from build123d import *

# Parameters (mm, degrees)
BOSS_EXTRUDE1_DEPTH      = 5.1
BOSS_EXTRUDE1_DEPTH_BACK = 5.1
SKETCH1_W                = 18
SKETCH1_H                = 15
SKETCH1_R                = 2.1
CUT_EXTRUDE1_DEPTH       = 4.1
CUT_EXTRUDE1_DEPTH_BACK  = 4.1
SKETCH4_W                = 6.8
SKETCH4_H                = 7.2
CUT_EXTRUDE2_DEPTH       = 7.5
SKETCH6_R                = 4.9
CUT_EXTRUDE4_DEPTH       = 4.5
SKETCH7_R                = 7.5
SKETCH7_R_2              = 3.225
BOSS_EXTRUDE2_DEPTH      = 1
SKETCH8_W                = 7.5
SKETCH8_H                = 2.6
CUT_EXTRUDE5_DEPTH       = 6.5


with BuildPart() as part:
    # Sketch1 → Boss-Extrude1 (new, two sides: drawn at the far end of the back side and taken through both)
    with BuildSketch(Plane(origin=(0, 0, 0), x_dir=(1, 0, 0), z_dir=(0, 1, 0)).offset(-BOSS_EXTRUDE1_DEPTH_BACK)):
        Rectangle(SKETCH1_W, SKETCH1_H)
        with Locations(Location((0, 0, 0), (0, 0, 270))):
            Circle(SKETCH1_R, mode=Mode.SUBTRACT)
    extrude(amount=BOSS_EXTRUDE1_DEPTH + BOSS_EXTRUDE1_DEPTH_BACK)

    # Sketch4 → Cut-Extrude1 (cut, two sides: drawn at the far end of the back side and taken through both)
    with BuildSketch(Plane(origin=(0, 0, 0), x_dir=(1, 0, 0), z_dir=(0, 1, 0)).offset(-CUT_EXTRUDE1_DEPTH_BACK)):
        Rectangle(SKETCH4_W, SKETCH4_H)
    extrude(amount=CUT_EXTRUDE1_DEPTH + CUT_EXTRUDE1_DEPTH_BACK, mode=Mode.SUBTRACT)

    # Sketch5 → Cut-Extrude2 (cut)
    with BuildSketch(Plane(origin=(0, 0, -7.5), x_dir=(-1, 0, 0), z_dir=(0, 0, -1))):
        Polygon((1.75, -0.4), (4.9, -0.4), (4.9, 4.1), (-4.9, 4.1), (-4.9, -0.4), (-1.75, -0.4), (-1.75, -4.1), (1.75, -4.1), align=None)
    extrude(amount=-CUT_EXTRUDE2_DEPTH, mode=Mode.SUBTRACT)

    # Sketch6 → Cut-Extrude4 (cut)
    with BuildSketch(Plane.XZ.offset(-4.1)):
        Circle(SKETCH6_R)
    extrude(amount=CUT_EXTRUDE4_DEPTH, mode=Mode.SUBTRACT)

    # Sketch7 → Boss-Extrude2 (add)
    with BuildSketch(Plane(origin=(0, 5.1, 0), x_dir=(1, 0, 0), z_dir=(0, 1, 0))):
        with Locations(Location((0, 0, 0), (0, 0, 270))):
            Circle(SKETCH7_R)
        with Locations(Location((0, 0, 0), (0, 0, 270))):
            Circle(SKETCH7_R_2, mode=Mode.SUBTRACT)
    extrude(amount=BOSS_EXTRUDE2_DEPTH)

    # Sketch8 → Cut-Extrude5 (cut)
    with BuildSketch(Plane.XY.offset(7.5)):
        with Locations((0, 1.65)):
            Rectangle(SKETCH8_W, SKETCH8_H)
    extrude(amount=-CUT_EXTRUDE5_DEPTH, mode=Mode.SUBTRACT)


solid = part.part
Here's how the part is built. I have some questions about the finished solid (model axes, mm). A direction names the side the tool comes from. Coordinates: 2 decimals unless noted, no trailing zeros. Write each loop counter-clockwise with the first axis right and the second up, starting at its lowest first coordinate (ties: lowest second). Pieces come first, ordered by that corner, then holes. Notation, with made-up numbers: (49.5, -32) - (103.5, -32) arc R7 cw to (103.5, -19) - close; hole circle Ø1 at (19.5, -6.5). An arc over 180 degrees is marked (long way). Use one line per item in the form item = value.
1) I need wall thicknesses on line 1 (X direction, y = 5.8, z = 0) (3 decimals); line 2 (Y direction, x = -0.75, z = -4.5); line 3 (Y direction, x = -0.25, z = -3). Which ranges of each line are inside material? Lowest first, please.
Solved:
line_1 = -7.5 to -3.225, 3.225 to 7.5
line_2 = -5.1 to -4.1, 4.1 to 6.1
line_3 = -5.1 to -4.1, 4.1 to 5.1
2) Suppose I cut it at C-C, the plane x = -2.5. Write out the boundary of the cut face in (y, z), plus the area to 3 significant figures.
Solved:
outline = (-5.1, -7.5) - (-0.4, -7.5) - (-0.4, -3.6) - (-4.1, -3.6) - (-4.1, 3.6) - (-0.4, 3.6) - (-0.4, 4.21) - (0.35, 4.21) - (0.35, 7.5) - (-5.1, 7.5) - close; (2.95, 4.21) - (4.1, 4.21) - (4.1, -7.5) - (5.1, -7.5) - (5.1, -7.07) - (6.1, -7.07) - (6.1, -2.04) - (5.1, -2.04) - (5.1, 2.04) - (6.1, 2.04) - (6.1, 7.07) - (5.1, 7.07) - (5.1, 7.5) - (2.95, 7.5) - close
area = 75.2 mm2
3) I'm going to push flat-ended pins straight in: P1, Ø6, axis at x = 0, z = 0, coming from the +Y side; P2, Ø2, axis at x = -0.5, y = -1, coming from the -Z side. Where does each tip first touch, or does it pass through?
Solved:
P1 = 5.1
P2 = 3.6
4) Thinking about a two-plate mould opening in Z: for faces 4 (the cylindrical face through (0.1, 0, 4.9)), 5 (the flat face through (3, -2, -3.6)), 6 (the cylindrical face through (0.631, 4.593, 2.003)), 7 (the flat face through (4.9, 2, -4)), which applies, released by +Z, released by -Z, zero draft, split by the parting line, or undercut?
Solved:
face_4 = released by -Z
face_5 = undercut
face_6 = undercut
face_7 = zero draft
5) Suppose I cut it at A-A, the plane x = 0.25. Give the number of separate pieces and of enclosed holes in the cut face, plus the area to 3 significant figures.
Solved:
separate_pieces = 4
enclosed_holes = 0
area = 49.6 mm2
6) On a 3-axis mill with a long thin cutter (end or side, diameter ignored), from which of +Z, -Z, +X, -X, +Y, -Y can I reach the whole of each face in a straight line? I mean faces 1 (the flat face through (0, 0.35, 6)), 2 (the flat face through (-3.4, -2, 0)), 3 (the flat face through (4, -0.4, -3)). Say none if no direction works.
Solved:
face_1 = +Z, -Z
face_2 = none
face_3 = -Z
7) Suppose I cut it at D-D, the plane y = 3.25. Write out the boundary of the cut face in (x, z), plus the area to 3 significant figures.
Solved:
outline = (-9, -7.5) - (-4.9, -7.5) - (-4.9, 0) arc R4.9 cw to (-3.4, 3.53) - (-3.4, 3.6) - (-3.32, 3.6) arc R4.9 cw to (3.32, 3.6) - (3.4, 3.6) - (3.4, 3.53) arc R4.9 cw to (4.9, 0) - (4.9, -7.5) - (9, -7.5) - (9, 7.5) - (-9, 7.5) - close
area = 159 mm2
8) Suppose I cut it at B-B, the plane z = 0.25. Write out the boundary of the cut face in (x, y).
Solved:
outline = (-9, -5.1) - (-2.09, -5.1) - (-2.09, -4.1) - (-3.4, -4.1) - (-3.4, -0.4) - (-4.89, -0.4) - (-4.89, 4.1) - (-2.09, 4.1) - (-2.09, 5.1) - (-3.22, 5.1) - (-3.22, 6.1) - (-7.5, 6.1) - (-7.5, 5.1) - (-9, 5.1) - close; (2.09, -5.1) - (9, -5.1) - (9, 5.1) - (7.5, 5.1) - (7.5, 6.1) - (3.22, 6.1) - (3.22, 5.1) - (2.09, 5.1) - (2.09, 4.1) - (4.89, 4.1) - (4.89, -0.4) - (3.4, -0.4) - (3.4, -4.1) - (2.09, -4.1) - close
